from build123d import *

# Parameters (mm, degrees)
EXTRUDE_1_DEPTH        = 1.5
HOLE_WIZARD_2_D        = 3.5
HOLE_WIZARD_4_D        = 1.5
PATTERN_LINEAR_2_COUNT = 4
PATTERN_LINEAR_2_PITCH = 5


with BuildPart() as part:
    # Эскиз1 → Вытянуть1 (new body)
    with BuildSketch(Plane(origin=(0, 0, 0), x_dir=(1, 0, 0), z_dir=(0, 1, 0))):
        with BuildLine():
            Line((-16, 41.5), (16, 41.5))
            Line((16, 41.5), (16, 3.5))
            Line((16, 3.5), (15, 3.5))
            ThreePointArc((15, 3.5), (13.939339828, 3.060660172), (13.5, 2))
            Line((13.5, 2), (13.5, -2))
            ThreePointArc((13.5, -2), (13.939339828, -3.060660172), (15, -3.5))
            Line((15, -3.5), (16, -3.5))
            Line((16, -3.5), (16, -41.5))
            Line((16, -41.5), (-16, -41.5))
            Line((-16, -41.5), (-16, -3.5))
            Line((-16, -3.5), (-15, -3.5))
            ThreePointArc((-15, -3.5), (-13.939339828, -3.060660172), (-13.5, -2))
            Line((-13.5, -2), (-13.5, 2))
            ThreePointArc((-13.5, 2), (-13.939339828, 3.060660172), (-15, 3.5))
            Line((-15, 3.5), (-16, 3.5))
            Line((-16, 3.5), (-16, 41.5))
        make_face()
    extrude(amount=EXTRUDE_1_DEPTH)

    # Отверстие2 (through all)
    with Locations(Plane(origin=(10.25, 1.5, -25.45), x_dir=(0, 0, 1), z_dir=(0, 1, 0))):
        with Locations((0, 0), (50.9, -20.5)):
            Hole(HOLE_WIZARD_2_D / 2)

    # Отверстие4 (through all)
    with Locations(Plane(origin=(9.68, 1.5, -38.5), x_dir=(0, 0, 1), z_dir=(0, 1, 0))):
        with Locations((0, 0), (77, 0)):
            hole_wizard_4 = Hole(HOLE_WIZARD_4_D / 2)

    # Линейный массив2: Отверстие4 ×4
    with Locations(*[(-i * PATTERN_LINEAR_2_PITCH, 0, 0) for i in range(1, PATTERN_LINEAR_2_COUNT)]):
        add(hole_wizard_4, mode=Mode.SUBTRACT)


solid = part.part
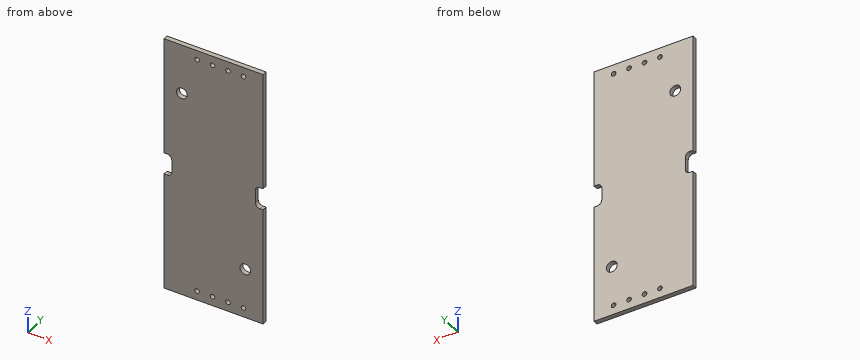
Read the model definition and answer for the solid it produces. Units are mm, in the model's axes. Round coordinates to 2 decimals unless told otherwise and drop trailing zeros. Write each loop counter-clockwise with the first axis right and the second up, starting at its lowest first coordinate (ties: lowest second). Pieces come first, ordered by that corner, then holes.
1. The part is cut by section D-D, the plane y = 1.25. State how many separate pieces and enclosed holes the cut face has, then the cut area to 3 significant figures.
2. Given pin 1 Ø0.8 at (y, z) = (1, 0) entering from -X, flat-ended and moving along its own axis, determine where the tip first touches the part or whether it passes through.
3. The part is cut by section B-B, the plane z = 38.5. Determine the outline of the cut face in (x, y), then the cut area to 3 significant figures.
4. The part is cut by section A-A, the plane z = 25.45. Determine the outline of the cut face in (x, y), then the cut area to 4 significant figures.
5. Straight lines are drawn through the part: L1, parallel to X at y = 1.1, z = 38.5; L2, parallel to Z at x = 10, y = 1.45; L3, parallel to Z at x = -14, y = 1.45. For each, find the intervals that lie inside material, in ascending order.
6. The part is cut by section C-C, the plane x = 4.68. Determine the outline of the cut face in (y, z), then the cut area to 3 significant figures.
Values:
1. separate pieces: 1
1. enclosed holes: 10
1. area: 2,590 mm2
2. pin 1: stops at x = -13.5
3. outline: (-16, 0) - (-6.07, 0) - (-6.07, 1.5) - (-16, 1.5) - close; (-4.57, 0) - (-1.07, 0) - (-1.07, 1.5) - (-4.57, 1.5) - close; (0.43, 0) - (3.93, 0) - (3.93, 1.5) - (0.43, 1.5) - close; (5.43, 0) - (8.93, 0) - (8.93, 1.5) - (5.43, 1.5) - close; (10.43, 0) - (16, 0) - (16, 1.5) - (10.43, 1.5) - close
3. area: 39.0 mm2
4. outline: (-16, 0) - (-12, 0) - (-12, 1.5) - (-16, 1.5) - close; (-8.5, 0) - (16, 0) - (16, 1.5) - (-8.5, 1.5) - close
4. area: 42.75 mm2
5. L1: x = -16 to -6.07, -4.57 to -1.07, 0.43 to 3.93, 5.43 to 8.93, 10.43 to 16
5. L2: z = -41.5 to -39.18, -37.82 to -27.18, -23.72 to 37.82, 39.18 to 41.5
5. L3: z = -41.5 to -3.12, 3.12 to 41.5
6. outline: (0, -41.5) - (1.5, -41.5) - (1.5, -39.25) - (0, -39.25) - close; (0, -37.75) - (1.5, -37.75) - (1.5, 37.75) - (0, 37.75) - close; (0, 39.25) - (1.5, 39.25) - (1.5, 41.5) - (0, 41.5) - close
6. area: 120 mm2
